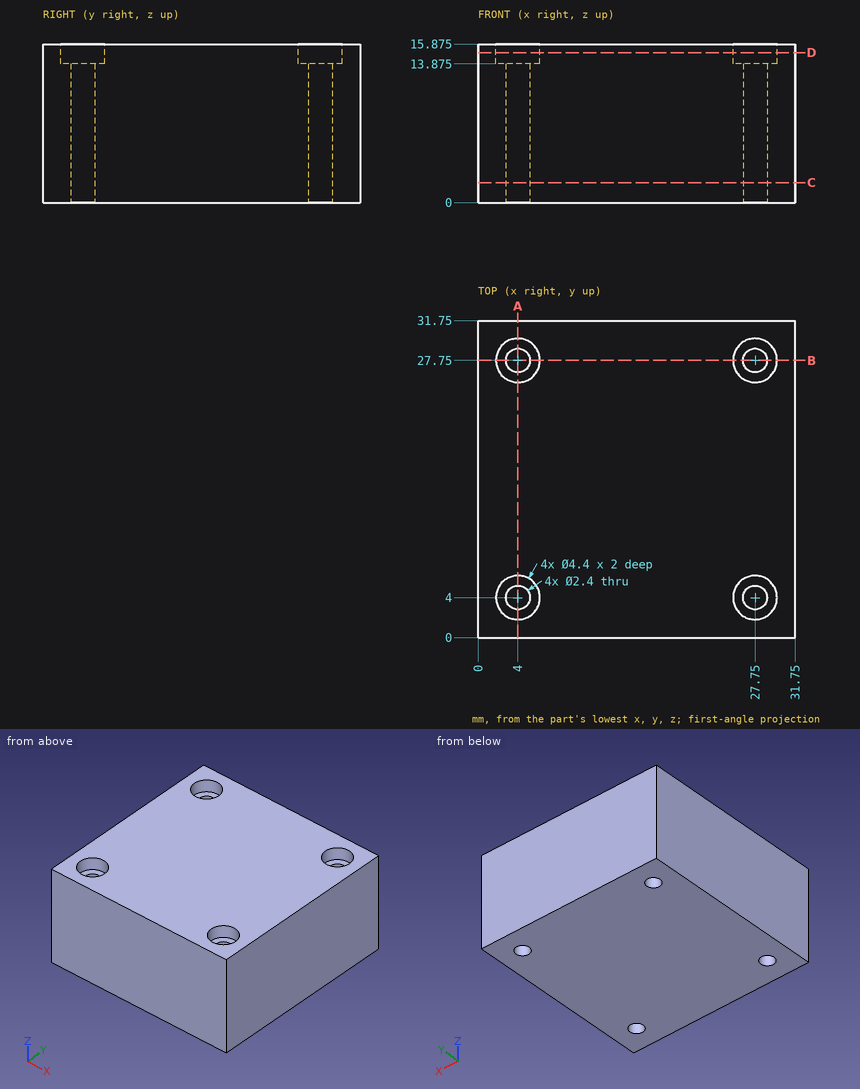
Design review of the part shown in the three views and the two pictorial views. Dimensions are in mm from the part's minimum x, y and z. Coordinates: 2 decimals unless noted, no trailing zeros. Write each loop counter-clockwise with the first axis right and the second up, starting at its lowest first coordinate (ties: lowest second). Pieces come first, ordered by that corner, then holes.
(1) Add section C-C on z = 2. Give the boundary of the cut face in (x, y), then the cut area to 3 significant figures.
(2) Add section D-D on z = 15. Give the boundary of the cut face in (x, y).
(3) For pin 1 Ø4 at (x, y) = (27.75, 27.75) entering from +Z (3 decimals), flat-tipped, find the tip position at first contact; note if it passes through.
(4) Wall thickness on probe 1 along Y at (x, z) = (27.75, 15.45); probe 2 along Y at (x, z) = (4, 3.5); probe 3 along X at (y, z) = (27, 9.75): over which ranges is each line inside the solid? List them lowest first.
(5) Add section A-A on x = 4. Give the boundary of the cut face in (y, z) (3 decimals), then the cut area to 3 significant figures.
Answer sheet:
1. outline: (0, 0) - (31.75, 0) - (31.75, 31.75) - (0, 31.75) - close; hole circle Ø2.4 at (4, 4); hole circle Ø2.4 at (4, 27.75); hole circle Ø2.4 at (27.75, 4); hole circle Ø2.4 at (27.75, 27.75)
1. area: 990 mm2
2. outline: (0, 0) - (31.75, 0) - (31.75, 31.75) - (0, 31.75) - close; hole circle Ø4.4 at (4, 4); hole circle Ø4.4 at (4, 27.75); hole circle Ø4.4 at (27.75, 4); hole circle Ø4.4 at (27.75, 27.75)
3. pin 1: stops at z = 13.875
4. probe 1: y = 0 to 1.8, 6.2 to 25.55, 29.95 to 31.75
4. probe 2: y = 0 to 2.8, 5.2 to 26.55, 28.95 to 31.75
4. probe 3: x = 0 to 3.06, 4.94 to 26.81, 28.69 to 31.75
5. outline: (0, 0) - (2.8, 0) - (2.8, 13.875) - (1.8, 13.875) - (1.8, 15.875) - (0, 15.875) - close; (5.2, 0) - (26.55, 0) - (26.55, 13.875) - (25.55, 13.875) - (25.55, 15.875) - (6.2, 15.875) - (6.2, 13.875) - (5.2, 13.875) - close; (28.95, 0) - (31.75, 0) - (31.75, 15.875) - (29.95, 15.875) - (29.95, 13.875) - (28.95, 13.875) - close
5. area: 420 mm2
